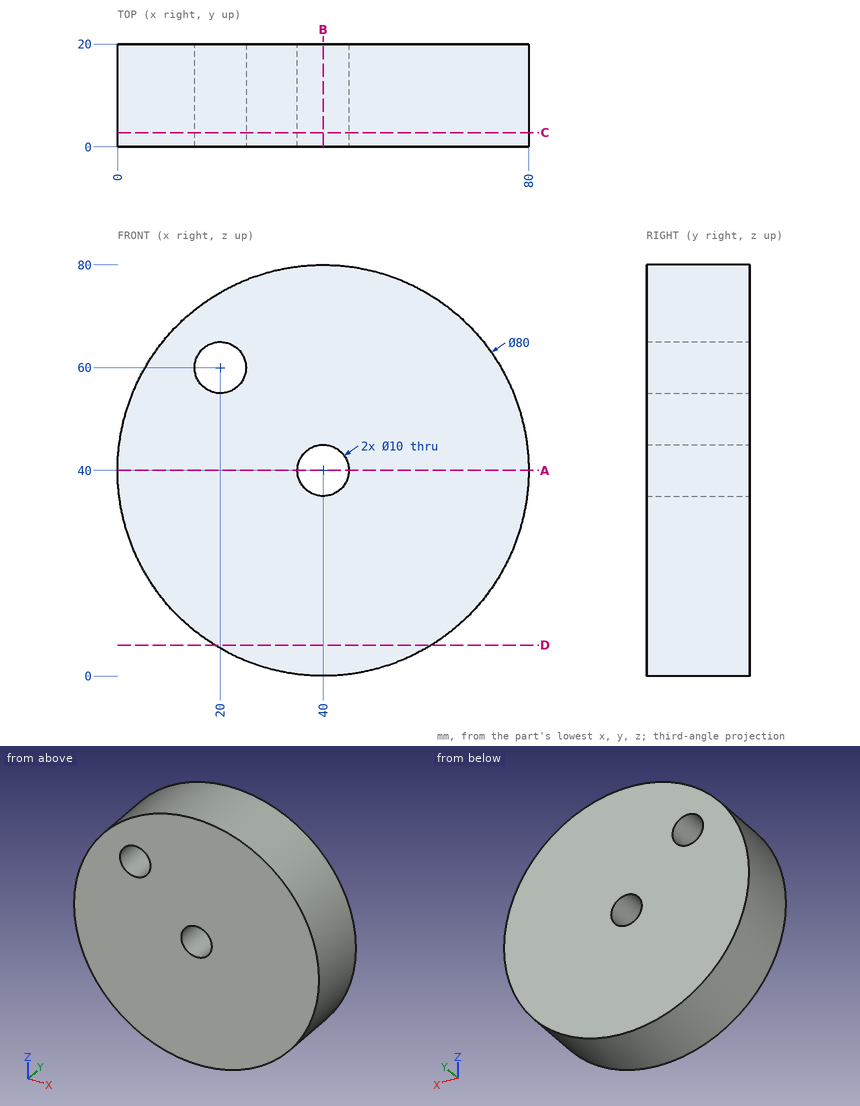
For this review, use the dimensioned drawing (mm, ordinates from the lowest corner) and the shaded views. Round coordinates to 2 decimals unless told otherwise and drop trailing zeros. Write each loop counter-clockwise with the first axis right and the second up, starting at its lowest first coordinate (ties: lowest second). Pieces come first, ordered by that corner, then holes. Notation, with made-up numbers: M -26.5,-1.75 L -22.5,-1.75 A21 ccw -22.5,23.25 Z; hole C -4,83.25 d7. An arc over 180 degrees is marked long. Answer as CSV lines item,"result". Start each with the question number.
Q1. Wall thickness on line 1 along Z through (x, y) = (40, 15); line 2 along X through (y, z) = (8.75, 60); line 3 along X through (y, z) = (16.75, 63): over which ranges is each line inside the solid? List them lowest first.
Q2. Consider section C-C, the plane y = 2.75. Give the boundary of the cut face in (x, z).
Q3. Clearance check with flat-ended pins moving along their axes: P1, Ø2, axis at x = 25.5, y = 7, coming from the -Z side; P2, Ø1, axis at x = 30, y = 7.5, coming from the +Z side; P3, Ø5, axis at x = 20.5, y = 11.5, coming from the -Z side; P4, Ø11.5, axis at x = 20, z = 60, coming from the +Y side. State where each tip first meets the part, or that it passes through.
Q4. Consider section D-D, the plane z = 6. Give the boundary of the cut face in (x, y), then the cut area to 3 significant figures.
Q5. Consider section B-B, the plane x = 40. Give the boundary of the cut face in (y, z).
Q6. Consider section A-A, the plane z = 40. Give the boundary of the cut face in (x, y), then the cut area to 3 significant figures.
Result set:
1,line 1,"z = 0 to 35, 45 to 80"
1,line 2,"x = 5.36 to 15, 25 to 74.64"
1,line 3,"x = 7.27 to 16, 24 to 72.73"
2,outline,"C 40,40 d80; hole C 20,60 d10; hole C 40,40 d10"
3,P1,"stops at z = 2.35"
3,P2,"stops at z = 78.86"
3,P3,"stops at z = 3.79"
3,P4,"stops at y = 20"
4,outline,"M 18.93,0 L 61.07,0 L 61.07,20 L 18.93,20 Z"
4,area,"843 mm²"
5,outline,"M 0,0 L 20,0 L 20,35 L 0,35 Z; M 0,45 L 20,45 L 20,80 L 0,80 Z"
6,outline,"M 0,0 L 35,0 L 35,20 L 0,20 Z; M 45,0 L 80,0 L 80,20 L 45,20 Z"
6,area,"1,400 mm²"
